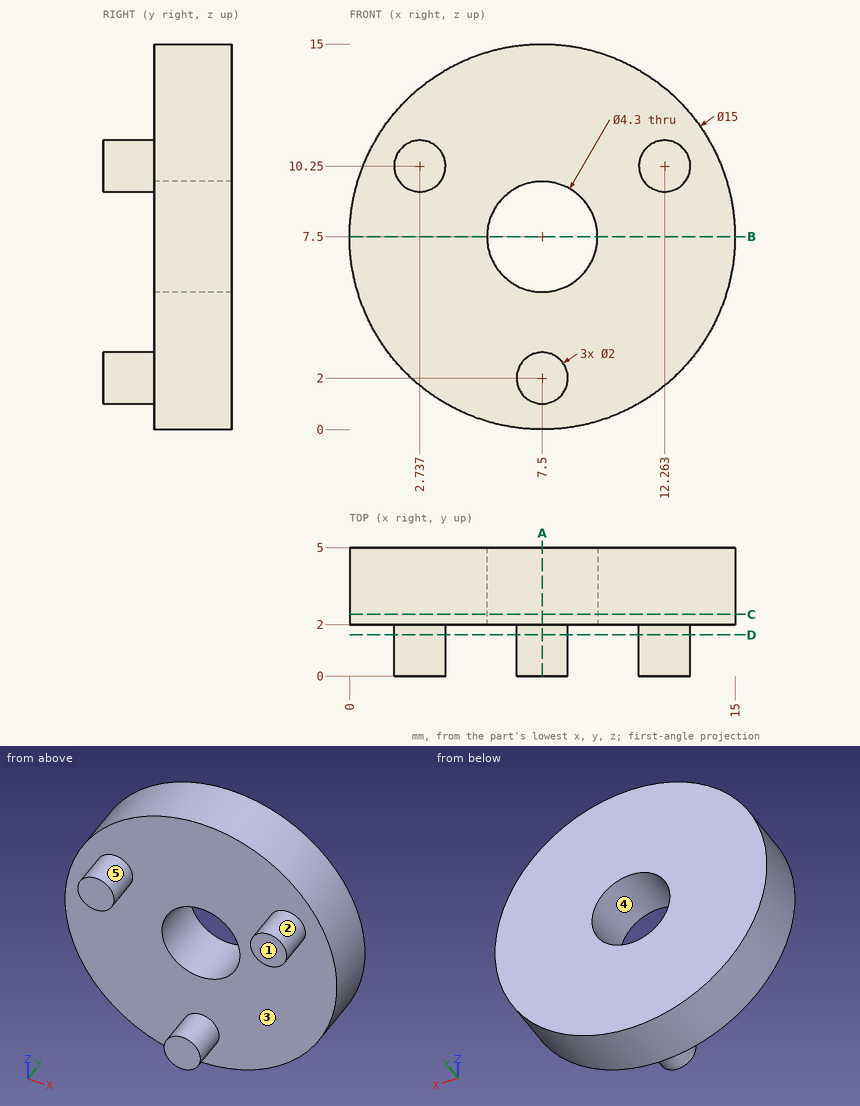
The drawing under review shows one solid part. Ordinate dimensions are in mm from its lowest x, y, z. A direction names the side the tool comes from. Round coordinates to 2 decimals unless told otherwise and drop trailing zeros. Loops run counter-clockwise (first coordinate to the right, second up) from the corner with the lowest first, then second, coordinate; pieces in that order, holes last. Notation, with made-up numbers: (33.5, 50) - (91.5, 50) arc R15 cw to (91.5, 73) - close; hole circle Ø5 at (-15.75, -37.5). An arc over 180 degrees is marked (long way). Use a Markdown table: item, result. Add a question column.
Q1. Add section A-A (x = 7.5). State the section outline as (y, z) points.
Q2. Add section C-C (y = 2.4). State the section outline as (x, z) points, plus the area to 3 significant figures.
Q3. Machinability: for the marked faces 1 and 2, which of the approach directions +Z, -Z, +X, -X, +Y, -Y give a long, thin tool a straight path to every point of the face, cutting with its end or side? Answer none if there is none.
Q4. Insertion check: pin 1 Ø1.5 at (x, z) = (2, 13) entering from -Y. The pin has a flat end and moves straight along its axis. Give the tip position at first contact, or say it passes through.
Q5. Add section D-D (y = 1.6). State the section outline as (x, z) points.
Q6. Add section B-B (z = 7.5). State the section outline as (x, y) points.
Q7. The part is to be moulded in two halves that separate along Z. For the marked faces 3, 4 and 5, say which applies: pulls with the +Z half, pulls with the -Z half, needs draft (parallel to the pull), parting line crosses it, or undercut.
Q8. For probe 1 along Y at (x, z) = (2.25, 11.25); probe 2 along X at (y, z) = (4.15, 7.75); probe 3 along Z at (x, y) = (13, 3), list the stretches that pass through material, from the lowest coordinate up.
Worked answers:
| question | item | result |
|---|---|---|
| 1 | outline | (0, 1) - (2, 1) - (2, 0) - (5, 0) - (5, 5.35) - (2, 5.35) - (2, 3) - (0, 3) - close; (2, 9.65) - (5, 9.65) - (5, 15) - (2, 15) - close |
| 2 | outline | circle Ø15 at (7.5, 7.5); hole circle Ø4.3 at (7.5, 7.5) |
| 2 | area | 162 mm² |
| 3 | face 1 | +Z, -Z, +X, -X, -Y |
| 3 | face 2 | -Y |
| 4 | pin 1 | y = 2 |
| 5 | outline | circle Ø2 at (2.74, 10.25); circle Ø2 at (7.5, 2); circle Ø2 at (12.26, 10.25) |
| 6 | outline | (0, 2) - (5.35, 2) - (5.35, 5) - (0, 5) - close; (9.65, 2) - (15, 2) - (15, 5) - (9.65, 5) - close |
| 7 | face 3 | needs draft |
| 7 | face 4 | undercut |
| 7 | face 5 | parting line crosses it |
| 8 | probe 1 | 2 to 5 |
| 8 | probe 2 | 0 to 5.36, 9.64 to 15 |
| 8 | probe 3 | 2.4 to 12.6 |
